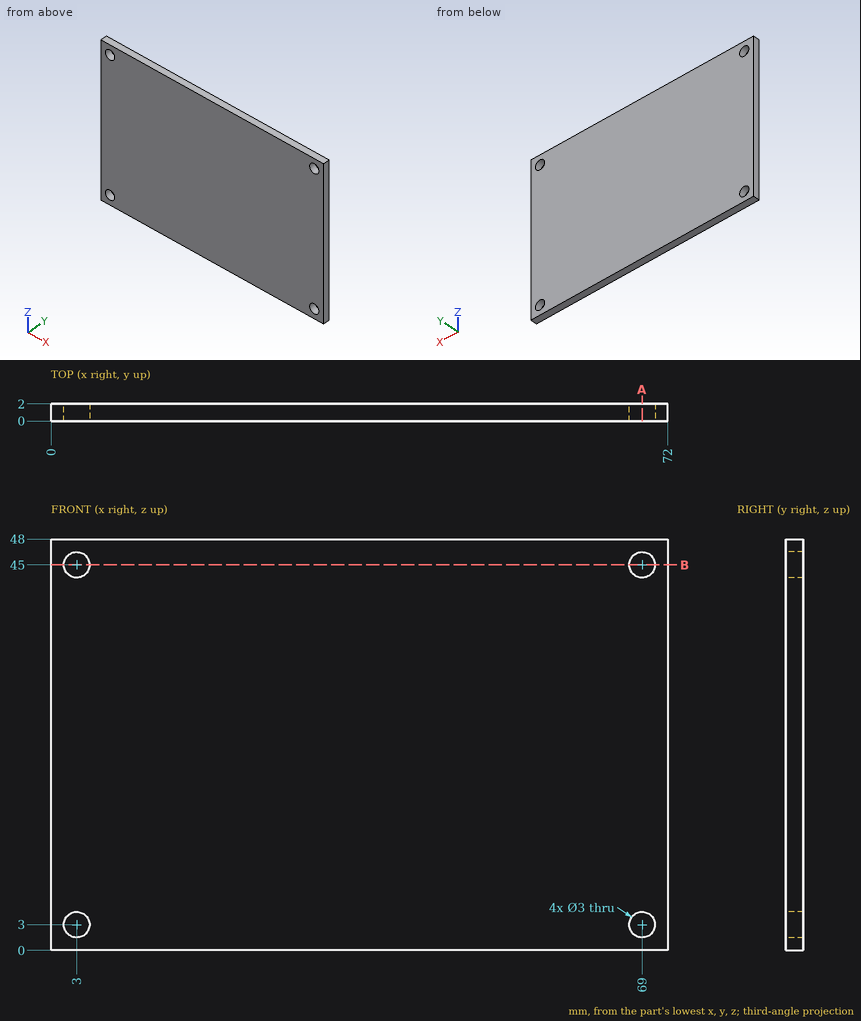
The figure shows three views and two pictorial views of one solid part (mm, origin at its lowest corner). Answer the questions. Round coordinates to 2 decimals unless told otherwise and drop trailing zeros. Write each loop counter-clockwise with the first axis right and the second up, starting at its lowest first coordinate (ties: lowest second). Pieces come first, ordered by that corner, then holes. Notation, with made-up numbers: M 68.25,38.25 L 122.25,38.25 A16 ccw 122.25,68.25 Z; hole C 33,11.5 d4. An arc over 180 degrees is marked long. Use a Markdown table: item, result.
1) The part is cut by section B-B (z = 45). Write down the section's boundary in (x, y).
Answers follow:
| item | result |
|---|---|
| outline | M 0,0 L 1.5,0 L 1.5,2 L 0,2 Z; M 4.5,0 L 67.5,0 L 67.5,2 L 4.5,2 Z; M 70.5,0 L 72,0 L 72,2 L 70.5,2 Z |
2) A flat-ended cylindrical pin translates along its axis: pin 1 (1.8 mm diameter, centred on x = 69, z = 45, fed in from -Y). Find the tip coordinate at first contact, or state that the pin passes through.
Answers follow:
| item | result |
|---|---|
| pin 1 | passes through |
3) The part is cut by section A-A (x = 69). Write down the section's boundary in (y, z), plus the area to 3 significant figures.
Answers follow:
| item | result |
|---|---|
| outline | M 0,0 L 2,0 L 2,1.5 L 0,1.5 Z; M 0,4.5 L 2,4.5 L 2,43.5 L 0,43.5 Z; M 0,46.5 L 2,46.5 L 2,48 L 0,48 Z |
| area | 84.0 mm2 |
4) Straight lines are drawn through the part: line 1 along Z through (x, y) = (69, 0.6); line 2 along X through (y, z) = (1.6, 4). For each, find the intervals that lie inside material, in ascending order. Write a range as [from, to].
Answers follow:
| item | result |
|---|---|
| line 1 | z = [0, 1.5], [4.5, 43.5], [46.5, 48] |
| line 2 | x = [0, 1.88], [4.12, 67.88], [70.12, 72] |
